Check sheet for the modelled part. Datum: model origin and axes. Units: mm. Coordinates: 2 decimals unless noted, no trailing zeros. Loops run counter-clockwise (first coordinate to the right, second up) from the corner with the lowest first, then second, coordinate; pieces in that order, holes last.
```python
from build123d import *

# Parameters (mm, degrees)
SKETCH021_R     = 1.5
PAD011_DEPTH    = 1.25
CHAMFER004_SIZE = 0.2


with BuildPart() as part:
    # Sketch021 → Pad011 (new body, symmetric)
    with BuildSketch(Plane.XY):
        Polygon((2.75, -1.5877132403), (2.75, 1.5877132403), (0, 3.1754264805), (-2.75, 1.5877132403), (-2.75, -1.5877132403), (0, -3.1754264805), align=None)
        Circle(SKETCH021_R, mode=Mode.SUBTRACT)
    extrude(amount=PAD011_DEPTH, both=True)

    # Sketch020 → Groove002 (revolve, cut)
    with BuildSketch(Plane.YZ):
        Polygon((-2.75, 1.25), (-3.5, 0.8169872981), (-3.5, 1.25), align=None)
        Polygon((-2.75, -1.25), (-3.5, -0.8169872981), (-3.5, -1.25), align=None)
    revolve(axis=Axis((0, 0, 0), (0, 0, 1)), mode=Mode.SUBTRACT)

    # Chamfer004
    chamfer004_edges = [part.edges().sort_by_distance(p)[0] for p in [
        (-1.5, 0, 1.25),
        (-1.5, 0, -1.25),
    ]]
    chamfer(chamfer004_edges, length=CHAMFER004_SIZE)


solid = part.part
```
1) Scan lines: line 1 (Y direction, x = -1.3, z = -0.25); line 2 (Y direction, x = -1, z = 0); line 3 (Y direction, x = 2.3, z = 0.05). Record each from-to range of solid material in increasing order.
Answer sheet:
line 1: y = -2.42 to -0.75, 0.75 to 2.42
line 2: y = -2.6 to -1.12, 1.12 to 2.6
line 3: y = -1.85 to 1.85
2) Section check A-A on z = -0.3. Enter the section's corners in (x, y).
Answer sheet:
outline: (-2.75, -1.59) - (0, -3.18) - (2.75, -1.59) - (2.75, 1.59) - (0, 3.18) - (-2.75, 1.59) - close; hole circle Ø3 at (0, 0)
3) Mould release check, pull along X, two halves, no side actions. Record for faces 1 (the cylindrical face through (-1.5, 0.07, -0.01)), 2 (the conical face through (-2.52, -1.44, 1.16)), 3 (the flat face through (1.36, -2.39, 0.02)), 4 (the flat face through (2, 0, 1.25)): +X half, -X half, draft (parallel to the pull), parting line (faces both ways), or undercut.
Answer sheet:
face 1: undercut
face 2: -X half
face 3: +X half
face 4: draft
4) Depth check by flat-ended pin: pin 1 (1 mm diameter, centred on x = 0.5, y = 1, fed in from +Z). Enter the tip coordinate at first touch or a pass-through.
Answer sheet:
pin 1: stops at z = 1.17
